Here's how the part is built. I have some questions about the finished solid (model axes, mm). Face numbers are marked on the shaded views. A direction names the side the tool comes from. Give positions to 0.01 mm unless a question says otherwise; leave off trailing zeros. Order: outer loops, then holes, each group sorted by start corner. A loop starts at its lowest first (then second) coordinate and runs counter-clockwise, first axis right, second up. Notation, with made-up numbers: M -7.75,43.5 L 40.25,43.5 A24 ccw 40.25,81.5 Z; hole C 8.5,62 d2. An arc over 180 degrees is marked long. Use CSV: the item, a comma, the result in double quotes. Start each with the question number.
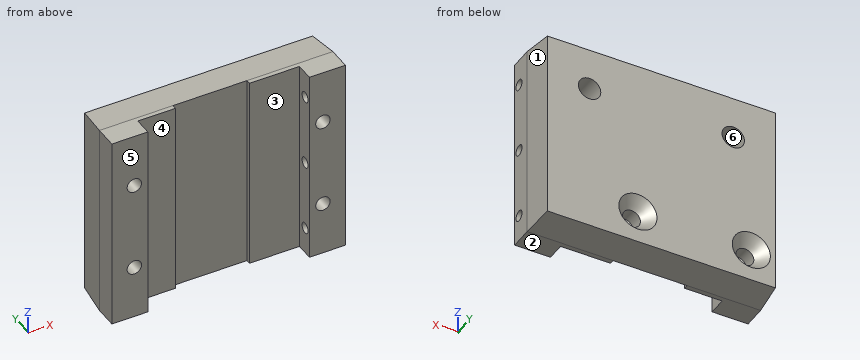
```python
from build123d import *

# Parameters (mm, degrees)
SKETCH1_W                             = 82.55
SKETCH1_H                             = 69.85
BOSS_EXTRUDE1_DEPTH                   = 7.9375
SKETCH2_W                             = 82.55
SKETCH2_H                             = 69.85
BOSS_EXTRUDE2_DEPTH                   = 3.175
F_3_8_16_TAPPED_HOLE1_D               = 7.9375
F_3_8_16_TAPPED_HOLE1_DEPTH           = 9.525
F_3_8_16_TAPPED_HOLE1_TIP             = 2.384665582
DRAFT1_ANGLE                          = 5
SKETCH3_W                             = 12.7
SKETCH3_H                             = 69.85
BOSS_EXTRUDE3_DEPTH                   = 7.9375
SKETCH4_W                             = 13.267261336
SKETCH4_H                             = 69.85
SKETCH4_W_2                           = 17.684109612
WEAR_PADS_DEPTH                       = 1.5875
F_10_24_TAPPED_HOLE1_D                = 3.7973
F_10_24_TAPPED_HOLE1_DEPTH            = 12.7
F_1_4_0_25_DIAMETER_HOLE1_D           = 6.35
F_1_4_0_25_DIAMETER_HOLE1_DEPTH       = 8.89
F_1_4_0_25_DIAMETER_HOLE1_CSINK_D     = 13.4874
F_1_4_0_25_DIAMETER_HOLE1_CSINK_ANGLE = 82
F_1_4_0_25_DIAMETER_HOLE1_TIP         = 1.907732465
F_1_4_20_TAPPED_HOLE1_D               = 5.1054
F_1_4_20_TAPPED_HOLE1_DEPTH           = 11.43
F_1_4_20_TAPPED_HOLE1_TIP             = 1.533816902
F_1_4_20_TAPPED_HOLE2_D               = 5.1054
F_1_4_20_TAPPED_HOLE2_DEPTH           = 11.43
F_1_4_20_TAPPED_HOLE2_TIP             = 1.533816902


with BuildPart() as part:
    # Sketch1 → Boss-Extrude1 (new body)
    with BuildSketch(Plane(origin=(0, 0, 0), x_dir=(1, 0, 0), z_dir=(0, 1, 0))):
        Rectangle(SKETCH1_W, SKETCH1_H)
    extrude(amount=BOSS_EXTRUDE1_DEPTH)

    # Sketch2 → Boss-Extrude2 (add)
    with BuildSketch(Plane(origin=(0, 7.9375, 0), x_dir=(1, 0, 0), z_dir=(0, 1, 0))):
        Rectangle(SKETCH2_W, SKETCH2_H)
    extrude(amount=BOSS_EXTRUDE2_DEPTH)

    # 3/8-16 Tapped Hole1
    with Locations(Plane(origin=(0, 11.1125, 0), x_dir=(1, 0, 0), z_dir=(0, 1, 0))):
        with Locations((-25.4, -19.05), (25.4, -19.05)):
            Hole(F_3_8_16_TAPPED_HOLE1_D / 2, depth=F_3_8_16_TAPPED_HOLE1_DEPTH)
            with Locations((0, 0, -(F_3_8_16_TAPPED_HOLE1_DEPTH + F_3_8_16_TAPPED_HOLE1_TIP / 2))):  # 118° drill point
                Cone(0, F_3_8_16_TAPPED_HOLE1_D / 2, F_3_8_16_TAPPED_HOLE1_TIP, mode=Mode.SUBTRACT)

    # Draft1
    draft1_faces = [part.faces().sort_by_distance(p)[0] for p in [
        (0, 5.55625, -34.925),
        (-41.275, 5.55625, 0),
        (0, 5.55625, 34.925),
        (41.275, 5.55625, 0),
    ]]
    draft(draft1_faces, Plane.ZX, DRAFT1_ANGLE)

    # Sketch3 → Boss-Extrude3 (add)
    with BuildSketch(Plane.XZ):
        with Locations((34.925, 0)):
            Rectangle(SKETCH3_W, SKETCH3_H)
        with Locations((-34.925, 0)):
            Rectangle(SKETCH3_W, SKETCH3_H)
    extrude(amount=BOSS_EXTRUDE3_DEPTH)

    # Sketch4 → Wear Pads (add)
    with BuildSketch(Plane.XZ):
        with Locations((-21.941369332, 0)):
            Rectangle(SKETCH4_W, SKETCH4_H)
        with Locations((19.732945194, 0)):
            Rectangle(SKETCH4_W_2, SKETCH4_H)
    extrude(amount=WEAR_PADS_DEPTH)

    # #10-24 Tapped Hole1
    with Locations(Plane(origin=(41.275, 0, 0), x_dir=(0, 0, -1), z_dir=(1, 0, 0))):
        with Locations((-25.4, -5.151627132), (25.4, -5.151627132), (0, -5.151627132)):
            Hole(F_10_24_TAPPED_HOLE1_D / 2, depth=F_10_24_TAPPED_HOLE1_DEPTH)

    # 1/4 (0.25) Diameter Hole1
    with Locations(Plane(origin=(0, 11.1125, 0), x_dir=(1, 0, 0), z_dir=(0, 1, 0))):
        with Locations((-31.795373704, 22.378883405), (8.300402943, 22.378883405)):
            CounterSinkHole(F_1_4_0_25_DIAMETER_HOLE1_D / 2, F_1_4_0_25_DIAMETER_HOLE1_CSINK_D / 2, depth=F_1_4_0_25_DIAMETER_HOLE1_DEPTH, counter_sink_angle=F_1_4_0_25_DIAMETER_HOLE1_CSINK_ANGLE)
            with Locations((0, 0, -(F_1_4_0_25_DIAMETER_HOLE1_DEPTH + F_1_4_0_25_DIAMETER_HOLE1_TIP / 2))):  # 118° drill point
                Cone(0, F_1_4_0_25_DIAMETER_HOLE1_D / 2, F_1_4_0_25_DIAMETER_HOLE1_TIP, mode=Mode.SUBTRACT)

    # 1/4-20 Tapped Hole1
    with Locations(Plane(origin=(0, -7.9375, 0), x_dir=(-1, 0, 0), z_dir=(0, -1, 0))):
        with Locations((-33.3375, 15.875), (-33.3375, -15.875)):
            Hole(F_1_4_20_TAPPED_HOLE1_D / 2, depth=F_1_4_20_TAPPED_HOLE1_DEPTH)
            with Locations((0, 0, -(F_1_4_20_TAPPED_HOLE1_DEPTH + F_1_4_20_TAPPED_HOLE1_TIP / 2))):  # 118° drill point
                Cone(0, F_1_4_20_TAPPED_HOLE1_D / 2, F_1_4_20_TAPPED_HOLE1_TIP, mode=Mode.SUBTRACT)

    # 1/4-20 Tapped Hole2
    with Locations(Plane(origin=(0, -7.9375, 0), x_dir=(-1, 0, 0), z_dir=(0, -1, 0))):
        with Locations((33.3375, -15.875), (33.3375, 15.875)):
            Hole(F_1_4_20_TAPPED_HOLE2_D / 2, depth=F_1_4_20_TAPPED_HOLE2_DEPTH)
            with Locations((0, 0, -(F_1_4_20_TAPPED_HOLE2_DEPTH + F_1_4_20_TAPPED_HOLE2_TIP / 2))):  # 118° drill point
                Cone(0, F_1_4_20_TAPPED_HOLE2_D / 2, F_1_4_20_TAPPED_HOLE2_TIP, mode=Mode.SUBTRACT)


solid = part.part
```
Q1. I need wall thicknesses on line 1 (X direction, y = 5, z = 19.05); line 2 (Y direction, x = 32.75, z = 25.4); line 3 (X direction, y = -5, z = -30.5) (3 decimals). Which ranges of each line are inside material? Lowest first, please. Write a range as [from, to].
Q2. Imagine slicing it at D-D, the plane x = 35. Count the separate pieces of the cut face and the enclosed holes in it, then the cut area to 3 significant figures.
Q3. We'd pull the mould along X, two halves only. Please class the marked faces 1, 2 and 3: pulls with the +X half, pulls with the -X half, needs draft (parallel to the pull), parting line crosses it, or undercut.
Q4. Imagine slicing it at C-C, the plane y = 8.75. Please give me the cut outline in (x, z).
Q5. Imagine slicing it at B-B, the plane x = 25.4. Please give me the cut outline in (y, z) (1 decimal), then the cut area to 3 significant figures.
Q6. Imagine slicing it at A-A, the plane z = 25.4. Please give me the cut outline in (x, y) (1 decimal).
Q7. For P1, Ø1.5, axis at y = 2.5, z = -24.5, coming from the +X side; P2, Ø8, axis at x = -6.5, z = 13.5, coming from the -Y side; P3, Ø8, axis at y = 8, z = 15.5, coming from the +X side; P4, Ø6.5, axis at x = 33.34, z = -15.88, coming from the -Y side, each with a flat end and sliding along its axis, tell me the tip position at first contact or that it passes through.
Q8. For the marked faces 4, 5 and 6, which set-ups out of +Z, -Z, +X, -X, +Y, -Y let a thin tool reach every point of the face, with its end or its side?
Reply:
1,line 1,"x = [-40.84, -29.37], [-21.43, 21.43], [29.37, 40.84]"
1,line 2,"y = [-7.94, -7.05], [-3.25, 11.11]"
1,line 3,"x = [-41.275, -28.575], [28.575, 41.275]"
2,separate pieces,"1"
2,enclosed holes,"3"
2,area,"1,190 mm^2"
3,face 1,"pulls with the +X half"
3,face 2,"needs draft"
3,face 3,"undercut"
4,outline,"M -40.51,-34.16 L 40.51,-34.16 L 40.51,34.16 L -40.51,34.16 Z; hole C -31.8,-22.38 d9.38; hole C -25.4,19.05 d7.94; hole C 8.3,-22.38 d9.38; hole C 25.4,19.05 d7.94"
5,outline,"M -1.6,-34.9 L 0,-34.9 L 11.1,-34 L 11.1,15.1 L 1.6,15.1 L 0,17.7 L 0,20.4 L 1.6,23 L 11.1,23 L 11.1,34 L 0,34.9 L -1.6,34.9 Z"
5,area,"792 mm^2"
6,outline,"M -41.3,-7.9 L -28.6,-7.9 L -28.6,-1.6 L -15.3,-1.6 L -15.3,0 L 10.9,0 L 10.9,-1.6 L 28.6,-1.6 L 28.6,-3.3 L 41.3,-3.3 L 41.3,0 L 40.3,11.1 L -40.3,11.1 L -41.3,0 Z; M 28.6,-7.9 L 41.3,-7.9 L 41.3,-7.1 L 28.6,-7.1 Z"
7,P1,"stops at x = 41.12"
7,P2,"stops at y = 0"
7,P3,"stops at x = 40.93"
7,P4,"stops at y = -7.94"
8,face 4,"+Z, -Z, -Y"
8,face 5,"+Z, -Z, +X, -X, -Y"
8,face 6,"+Y"
